Read the model definition and answer for the solid it produces. Units are mm, in the model's axes. Face numbers are marked on the shaded views. Coordinates: 2 decimals unless noted, no trailing zeros. Loops run counter-clockwise (first coordinate to the right, second up) from the corner with the lowest first, then second, coordinate; pieces in that order, holes last. Notation, with made-up numbers: (6, 25.25) -> (14, 25.25) arc R5 cw to (14, 31.25) -> close; hole circle Ø2 at (-22, -1). An arc over 180 degrees is marked (long way). One line per question, with ' | ' between items. Start each with the question number.
Autodesk Inventor part; units mm, degrees
ref_plane "YZ Plane" through (0, 0, 0) normal (1, 0, 0) x (0, 1, 0)
ref_plane "XZ Plane" through (0, 0, 0) normal (0, 1, 0) x (-1, 0, 0)
ref_plane "XY Plane" through (0, 0, 0) normal (0, 0, 1) x (1, 0, 0)
sketch "Skizze1" plane through (0, 0, 0) normal (0, 1, 0) x (-1, 0, 0)
  line L0 (35.25, -25.25) -> (-35.25, -25.25)
  line L1 (-35.25, -25.25) -> (-35.25, 25.25)
  line L2 (-35.25, 25.25) -> (35.25, 25.25)
  line L3 (35.25, 25.25) -> (35.25, -25.25)
  line L4 (35.25, -25.25) -> (-35.25, 25.25) construction
  line L5 (-35.25, -25.25) -> (35.25, 25.25) construction
  line L6 (37.65, -27.65) -> (-37.65, -27.65)
  line L7 (-37.65, -27.65) -> (-37.65, 27.65)
  line L8 (-37.65, 27.65) -> (37.65, 27.65)
  line L9 (37.65, 27.65) -> (37.65, -27.65)
  line L10 (32.85, -22.85) -> (-32.85, -22.85)
  line L11 (-32.85, -22.85) -> (-32.85, 22.85)
  line L12 (-32.85, 22.85) -> (32.85, 22.85)
  line L13 (32.85, 22.85) -> (32.85, -22.85)
  line L14 (47.65, -27.65) -> (37.65, -27.65)
  line L15 (37.65, 27.65) -> (47.65, 27.65)
  circle A0 centre (47.65, 0) radius 2
  line L16 (-37.65, -27.65) -> (-47.65, -27.65)
  line L17 (-37.65, 27.65) -> (-47.65, 27.65)
  circle A1 centre (-47.65, 0) radius 2
  arc A2 (-47.65, 27.65) -> (-57.65, 17.65) centre (-47.65, 17.65) ccw
  arc A3 (-57.65, -17.65) -> (-47.65, -27.65) centre (-47.65, -17.65) ccw
  line L18 (-57.65, 17.65) -> (-57.65, -17.65)
  arc A4 (57.65, 17.65) -> (47.65, 27.65) centre (47.65, 17.65) ccw
  arc A5 (47.65, -27.65) -> (57.65, -17.65) centre (47.65, -17.65) ccw
  line L19 (57.65, 17.65) -> (57.65, -17.65)
  point P0 (0, 0)
  point P1 (86.5572, 0)
  point P2 (-87.7335, 0)
  point P3 (57.65, 0)
  point P4 (-57.65, 0)
  dimension "d0" = 70.5
  dimension "d1" = 50.5
  dimension "d2" = 2.4
  dimension "d3" = 2.4
  dimension "d4" = 4
  dimension "d7" = 4
  dimension "d28" = 20
  dimension "d29" = 20
  dimension "d30" = 10
  dimension "d31" = 10
  dimension "d32" = 10
  dimension "d33" = 10
extrude "Extrusion1" add sketch "Skizze1" against normal blind 2 contours L0 L1 L2 L3 | L6 L7 L8 L9 | L9 L15 A4 L19 A5 L14 | L16 A3 L18 A2 L17 L7 | L10 L11 L12 L13
extrude "Extrusion2" add sketch "Skizze1" along normal blind 5 contours L6 L7 L8 L9 | L9 L15 A4 L19 A5 L14 | L16 A3 L18 A2 L17 L7
extrude "Extrusion3" add sketch "Skizze1" along normal blind 2 contours L0 L1 L2 L3
sketch "Skizze2" plane through (0, 0, 0) normal (0, 0, 1) x (1, 0, 0)
  line L0 (32.85, 0) -> (32.85, 2)
  line L1 (32.85, 2) -> (35.25, 2)
  line L2 (35.25, 2) -> (35.25, 5)
  line L3 (35.25, 5) -> (45.65, 5)
  line L4 (45.65, 5) -> (45.65, -2)
  line L5 (45.65, -2) -> (-45.65, -2)
  line L6 (-45.65, -2) -> (-45.65, 5)
  line L7 (-45.65, 5) -> (-35.25, 5)
  line L8 (-35.25, 5) -> (-35.25, 2)
  line L9 (-35.25, 2) -> (-32.85, 2)
  line L10 (-32.85, 2) -> (-32.85, 0)
  line L11 (-32.85, 0) -> (32.85, 0)
  line L12 (-57.65, 5) -> (-49.65, 5)
  line L13 (-49.65, 5) -> (-49.65, -2)
  line L14 (-49.65, -2) -> (-57.65, -2)
  line L15 (49.65, 5) -> (57.65, 5)
  line L16 (57.65, -2) -> (49.65, -2)
  line L17 (49.65, -2) -> (49.65, 5)
  arc A0 (-35.25, 3.5) -> (-35.25, 5) centre (-35.25, 4.25) ccw
  arc A1 (35.25, 5) -> (35.25, 3.5) centre (35.25, 4.25) ccw
  line L18 (-35.25, 5) -> (-35.25, 3.5)
  line L19 (35.25, 5) -> (35.25, 3.5)
  line L20 (-34.5, 4.25) -> (-34.5, 3.5)
  line L21 (-35.25, 2) -> (35.25, 2)
  line L22 (35.25, 2) -> (35.25, 5)
  line L23 (-35.25, 3.5) -> (35.25, 3.5)
  line L24 (-35.25, 5) -> (35.25, 5)
  line L25 (47.65, 5) -> (-47.65, 5)
  line L26 (34.5, 4.25) -> (34.5, 3.5)
  line L27 (-57.65, -2) -> (-57.65, 5)
  line L28 (57.65, 5) -> (57.65, -2)
  point P0 (0, 0)
  point P1 (39.5, 3.725)
  point P2 (39.8372, 3.6239)
  point P3 (-39.5, 3.725)
  point P4 (-39.8372, 3.6239)
  dimension "d14" = 1.5
  dimension "d15" = 1.5
extrude "Extrusion4" add sketch "Skizze2" along normal mid plane 50.5 contours A1 L2 | L8 A0
extrude "Extrusion5" cut sketch "Skizze2" along normal through all both and the other way through all contours A1 L26 L23 L20 A0 L24
sketch "Skizze3" plane through (0, 5, 0) normal (0, 1, 0) x (1, 0, 0)
  circle A0 centre (-47.65, 0) radius 2
  circle A1 centre (47.65, 0) radius 2
  point P0 (0, 0)
hole "Bohrung1" at (-47.65, 5, 0) at (47.65, 5, 0) direction (0, -1, 0) diameter 4.5 depth 6 countersink diameter 9.4 countersink angle 90
equation "\"d7\" = d4"
equation "\"d29\" = d28"
equation "\"d32\" = d31"
equation "\"d33\" = d30"
equation "\"d15\" = d14"
properties part number "PCB_Holder_B"
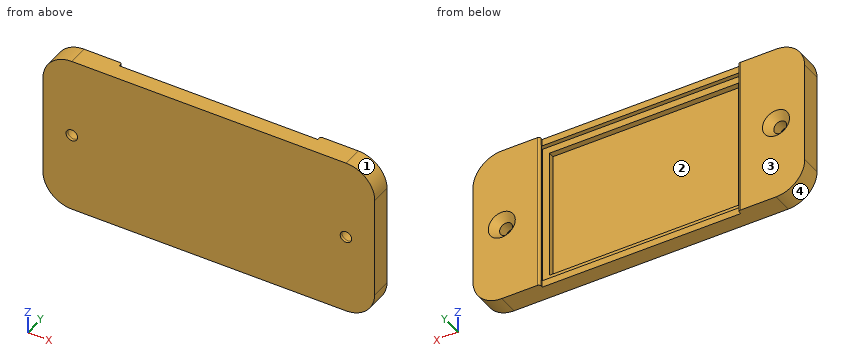
(1) Find the intervals of material crossed by probe 1 along X at (y, z) = (0.3, 0); probe 2 along X at (y, z) = (-1.4, 0); probe 3 along Z at (x, y) = (-47.65, 0.35), in increasing order. Write a range as from..to.
(2) Determine the mould class of the marked faces 1, 2, 3 and 4 for opening direction X: +X half, -X half, draft (parallel to the pull), parting line (faces both ways), or undercut.
(3) Section A-A on x = 11 is taken. Write down the section's boundary in (y, z).
(4) Each of these flat-tipped pins is pushed along its axis until it touches: pin 1 Ø5 at (x, z) = (-47.65, 0) entering from +Y; pin 2 Ø4.5 at (x, z) = (47.65, 0) entering from -Y; pin 3 Ø0.6 at (y, z) = (4, 26.5) entering from -X; pin 4 Ø3 at (x, z) = (-15, -14.5) entering from +Y. Where does it stop, or does it pass through?
(5) Section B-B on z = 7.5 is taken. Write down the section's boundary in (x, y).
Working result:
1) probe 1: x = -57.65..-49.9, -45.4..-32.85, 32.85..45.4, 49.9..57.65 | probe 2: x = -57.65..-49.65, -45.65..45.65, 49.65..57.65 | probe 3: z = -27.65..-2.25, 2.25..27.65
2) face 1: +X half | face 2: undercut | face 3: draft | face 4: -X half
3) outline: (-2, -27.65) -> (3.5, -27.65) -> (3.5, -25.25) -> (2, -25.25) -> (2, -22.85) -> (0, -22.85) -> (0, 22.85) -> (2, 22.85) -> (2, 25.25) -> (3.5, 25.25) -> (3.5, 27.65) -> (-2, 27.65) -> close
4) pin 1: stops at y = 2.8 | pin 2: stops at y = -2 | pin 3: stops at x = -52.84 | pin 4: stops at y = 0
5) outline: (-57.65, -2) -> (57.65, -2) -> (57.65, 5) -> (35.25, 5) arc R0.75 ccw to (35.25, 3.5) -> (35.25, 2) -> (32.85, 2) -> (32.85, 0) -> (-32.85, 0) -> (-32.85, 2) -> (-35.25, 2) -> (-35.25, 3.5) arc R0.75 ccw to (-35.25, 5) -> (-57.65, 5) -> close
